Could you check a few things on this model? Use its own coordinates, in mm. A direction names the side the tool comes from. Give positions to 0.01 mm unless a question says otherwise; leave off trailing zeros. Order: outer loops, then holes, each group sorted by start corner. A loop starts at its lowest first (then second) coordinate and runs counter-clockwise, first axis right, second up. Notation, with made-up numbers: (11.5, 46) -> (65.5, 46) arc R8 cw to (65.5, 53) -> close; hole circle Ø5 at (26, -18.5). An arc over 180 degrees is marked (long way). Answer as CSV lines item,"result". Start each with the question number.
(1) I want a section at B-B (x = 92). Please give me the cut outline in (y, z), plus the area to 3 significant figures.
(2) Will these pins go through, and if not, where does the flat tip stop? pin 1 Ø5 at (x, y) = (79.5, 55.5) entering from -Z; pin 2 Ø12 at (x, y) = (-41.5, 65.5) entering from +Z.
(3) I want a section at C-C (z = 29.5). Please give me the cut outline in (x, y), plus the area to 3 significant figures.
(4) I want a section at A-A (y = -39). Please give me the cut outline in (x, z).
(5) On a 3-axis mill with a long thin cutter (end or side, diameter ignored), from which of +Z, -Z, +X, -X, +Y, -Y can I reach the whole of each face in a straight line? I mean faces 1 (the face through (99, -2, 57)), 2 (the face through (115, -2, 49)). Say none if no direction works.
(6) I need wall thicknesses on L1, parallel to X at y = -11, z = 88; L2, parallel to Z at x = 27, y = -89. Which ranges of each line are inside material? Lowest first, please.
```python
from build123d import *

# Parameters (mm, degrees)
SKETCH_1_W             = 230
SKETCH_1_H             = 240
EXTRUDE_1_DEPTH        = 16
SKETCH_3_R             = 13
CUT_EXTRUDE_1_DEPTH    = 167.976046186
PATTERN_LINEAR_1_COUNT = 3
PATTERN_LINEAR_1_PITCH = 80
SKETCH_4_W             = 16
SKETCH_4_H             = 240
EXTRUDE_2_DEPTH        = 84
SKETCH_5_R             = 13
CUT_EXTRUDE_2_DEPTH    = 265.945277369
PATTERN_LINEAR_2_COUNT = 3
PATTERN_LINEAR_2_PITCH = 80
SKETCH_6_W             = 214
SKETCH_6_H             = 240
EXTRUDE_3_DEPTH        = 16
SKETCH_7_W             = 84
SKETCH_7_H             = 240
EXTRUDE_4_DEPTH        = 16


with BuildPart() as part:
    # 草图1 → 凸台-拉伸1 (new body)
    with BuildSketch(Plane.XY):
        Rectangle(SKETCH_1_W, SKETCH_1_H)
    extrude(amount=EXTRUDE_1_DEPTH)

    # 草图3 → 切除-拉伸1 (cut, through all)
    with BuildSketch(Plane.XY.offset(16)):
        with Locations((-73, 80)):
            Circle(SKETCH_3_R)
        with Locations((-14.5, 80)):
            Circle(SKETCH_3_R)
        with Locations((43.5, 80)):
            Circle(SKETCH_3_R)
    cut_extrude_1 = extrude(amount=-CUT_EXTRUDE_1_DEPTH, mode=Mode.SUBTRACT)

    # 阵列(线性)1: 切除-拉伸1 ×3
    with Locations(*[(0, -i * PATTERN_LINEAR_1_PITCH, 0) for i in range(1, PATTERN_LINEAR_1_COUNT)]):
        add(cut_extrude_1, mode=Mode.SUBTRACT)

    # 草图4 → 凸台-拉伸2 (add)
    with BuildSketch(Plane.XY.offset(16)):
        with Locations((107, 0)):
            Rectangle(SKETCH_4_W, SKETCH_4_H)
    extrude(amount=EXTRUDE_2_DEPTH)

    # 草图5 → 切除-拉伸2 (cut, through all)
    with BuildSketch(Plane.ZY.offset(-99)):
        with Locations((48, 80)):
            Circle(SKETCH_5_R)
    cut_extrude_2 = extrude(amount=-CUT_EXTRUDE_2_DEPTH, mode=Mode.SUBTRACT)

    # 阵列(线性)2: 切除-拉伸2 ×3
    with Locations(*[(0, -i * PATTERN_LINEAR_2_PITCH, 0) for i in range(1, PATTERN_LINEAR_2_COUNT)]):
        add(cut_extrude_2, mode=Mode.SUBTRACT)

    # 草图6 → 凸台-拉伸3 (add)
    with BuildSketch(Plane.XY.offset(16)):
        with Locations((-8, 0)):
            Rectangle(SKETCH_6_W, SKETCH_6_H)
    extrude(amount=-EXTRUDE_3_DEPTH)

    # 草图7 → 凸台-拉伸4 (add)
    with BuildSketch(Plane.ZY.offset(-99)):
        with Locations((58, 0)):
            Rectangle(SKETCH_7_W, SKETCH_7_H)
    extrude(amount=-EXTRUDE_4_DEPTH)


solid = part.part
```
Final values:
1,outline,"(-120, 0) -> (120, 0) -> (120, 16) -> (-120, 16) -> close"
1,area,"3,840 mm²"
2,pin 1,"z = 0"
2,pin 2,"z = 16"
3,outline,"(99, -120) -> (115, -120) -> (115, 120) -> (99, 120) -> close"
3,area,"3,840 mm²"
4,outline,"(-115, 0) -> (115, 0) -> (115, 100) -> (99, 100) -> (99, 16) -> (-115, 16) -> close"
5,face 1,"+Z, -X, +Y, -Y"
5,face 2,"+Z, -Z, +X, +Y, -Y"
6,L1,"99 to 115"
6,L2,"0 to 16"
